Part model, mm, in its own coordinate system. A direction names the side the tool comes from. Round coordinates to 2 decimals unless told otherwise and drop trailing zeros. Write each loop counter-clockwise with the first axis right and the second up, starting at its lowest first coordinate (ties: lowest second). Pieces come first, ordered by that corner, then holes.
```python
from build123d import *

# Parameters (mm, degrees)
F2_DEPTH  = 152.4
F3_W      = 1.27
F3_H      = 2.54
F4_DEPTH  = 126.6662840818
F8_DEPTH  = 1.27
F12_DEPTH = 1.27


# Not quite as in the source:
# - the program builds the solid bodies; features that only make, move or delete a surface that nothing else refers to are left out


with BuildPart() as f2:
    # F1 (on Top) → F2 (new body)
    with BuildSketch(Plane.XY):
        Polygon((-9.144, 0), (53.5142840818, 0), (53.5142840818, -84.328), (0, -84.328), (0, -96.0219023137), (53.5142840818, -96.0219023137), (71.9958739355, -96.0219023137), (71.9958739355, 33.6619690061), (53.5142840818, 33.6619690061), (-9.144, 33.6619690061), align=None)
    extrude(amount=F2_DEPTH)

    # F3 (on face) → F4 (join, through all)
    with BuildSketch(Plane(origin=(53.5142840818, 0, 0), x_dir=(0, -1, 0), z_dir=(-1, 0, 0))):
        with Locations((0.635, 74.93)):
            Rectangle(F3_W, F3_H)
        with Locations((83.693, 74.93)):
            Rectangle(F3_W, F3_H)
        with Locations((44.1576857662, 74.93)):
            Rectangle(F3_W, F3_H)
    extrude(amount=F4_DEPTH)

    # F7 (on face) → F8 (join)
    with BuildSketch(Plane.XZ):
        Polygon((-4.7359238379, 104.818597436), (-73.152, 76.2), (-66.5699955492, 76.2), (-4.7359238379, 102.0653302762), align=None)
    extrude(amount=F8_DEPTH)

    # F11 (on face) → F12 (join)
    with BuildSketch(Plane(origin=(0, -84.328, 0), x_dir=(-1, 0, 0), z_dir=(0, 1, 0))):
        Polygon((-5.7641793689, 106.457546895), (9.144, 100.221422174), (66.5699955492, 76.2), (73.152, 76.2), (9.144, 102.9746893338), (-5.7641793689, 109.2108140547), align=None)
    extrude(amount=F12_DEPTH)


solid = f2.part
```
Q1. Cut at C-C on y = -76. Write the cut outline in (x, z), plus the area to 3 significant figures.
Values follow:
outline: (53.51, 0) - (72, 0) - (72, 152.4) - (53.51, 152.4) - close
area: 2,820 mm2
Q2. Wall check: L1, parallel to Y at x = 31, z = 35; L2, parallel to X at y = 27.5, z = 79.5; L3, parallel to X at y = -20.5, z = 50.5. Give the ranges that are in metal, low to high.
Values follow:
L1: y = -96.02 to -84.33, 0 to 33.66
L2: x = -9.14 to 72
L3: x = 53.51 to 72
Q3. Mould opens along Y. For faces 1 (the flat face through (35, -96.022, 75)), 2 (the flat face through (53.514, -42, 75)), 3 (the flat face through (-36.09, -0.63, 88.95)) say: +Y half, -Y half, draft (parallel to the pull), parting line (faces both ways), or undercut.
Values follow:
face 1: -Y half
face 2: undercut
face 3: draft
Q4. Cut at B-B on z = 64.5. Write the cut outline in (x, y).
Values follow:
outline: (-9.14, 0) - (53.51, 0) - (53.51, -84.33) - (0, -84.33) - (0, -96.02) - (72, -96.02) - (72, 33.66) - (-9.14, 33.66) - close
Q5. Drop flat-ended pins along their axis: pin 1 (5 mm diameter, centred on y = -63.5, z = 59.5, fed in from -X); pin 2 (13 mm diameter, centred on y = -93, z = 64, fed in from -X); pin 3 (0.6 mm diameter, centred on x = 1, y = -83.5, fed in from -Z); pin 4 (9.5 mm diameter, centred on x = -33, z = 82.5, fed in from -Y). Give the stop position or say it passes through.
Values follow:
pin 1: stops at x = 53.51
pin 2: stops at x = 0
pin 3: stops at z = 73.66
pin 4: passes through
Q6. Cut at A-A on x = -20.5. Write the cut outline in (y, z), plus the area to 3 significant figures.
Values follow:
outline: (-84.33, 73.66) - (-83.06, 73.66) - (-83.06, 76.2) - (-84.33, 76.2) - close; (-84.33, 95.47) - (-83.06, 95.47) - (-83.06, 98.22) - (-84.33, 98.22) - close; (-44.79, 73.66) - (-43.52, 73.66) - (-43.52, 76.2) - (-44.79, 76.2) - close; (-1.27, 73.66) - (0, 73.66) - (0, 76.2) - (-1.27, 76.2) - close; (-1.27, 95.47) - (0, 95.47) - (0, 98.22) - (-1.27, 98.22) - close
area: 16.7 mm2
Q7. Which spindle directions (+Z, -Z, +X, -X, +Y, -Y) get a long thin tool onto all of the face, cutting with end or side? Do faces 4 (the flat face through (-41.3, 0, 87.3)), 5 (the flat face through (32, 33.662, 75)), 6 (the flat face through (-36.4, -84.328, 89.1)), 7 (the flat face through (-19, -1.27, 75)), 8 (the flat face through (22, 0, 36)). Say none if no direction does.
Values follow:
face 4: +Z, -Z, -X, +Y
face 5: +Z, -Z, +X, -X, +Y
face 6: +Z, -Z, -X, -Y
face 7: +Z, -Z, -X
face 8: -Z, -X
